```python
from build123d import *

# Parameters (mm, degrees)
SKETCH1_W           = 40
SKETCH1_H           = 40
BOSS_EXTRUDE1_DEPTH = 40
SKETCH2_W           = 10
SKETCH2_H           = 20
CUT_EXTRUDE1_DEPTH  = 40
SKETCH3_W           = 10
SKETCH3_H           = 10
CUT_EXTRUDE2_DEPTH  = 40
SKETCH4_W           = 10
SKETCH4_H           = 10
CUT_EXTRUDE4_DEPTH  = 20
SKETCH5_W           = 10
SKETCH5_H           = 10
CUT_EXTRUDE5_DEPTH  = 30


with BuildPart() as part:
    # Sketch1 → Boss-Extrude1 (new body)
    with BuildSketch(Plane.XY):
        with Locations((20, 20)):
            Rectangle(SKETCH1_W, SKETCH1_H)
    extrude(amount=BOSS_EXTRUDE1_DEPTH)

    # Sketch2 → Cut-Extrude1 (cut)
    with BuildSketch(Plane(origin=(0, 40, 0), x_dir=(1, 0, 0), z_dir=(0, 1, 0))):
        with Locations((35, -30)):
            Rectangle(SKETCH2_W, SKETCH2_H)
    extrude(amount=-CUT_EXTRUDE1_DEPTH, mode=Mode.SUBTRACT)

    # Sketch3 → Cut-Extrude2 (cut)
    with BuildSketch(Plane.ZY):
        with Locations((25, 35)):
            Rectangle(SKETCH3_W, SKETCH3_H)
        Polygon((40, 10), (40, 40), (30, 40), (30, 30), (30, 10), align=None)
    extrude(amount=-CUT_EXTRUDE2_DEPTH, mode=Mode.SUBTRACT)

    # Sketch4 → Cut-Extrude4 (cut)
    with BuildSketch(Plane(origin=(0, 30, 0), x_dir=(1, 0, 0), z_dir=(0, 1, 0))):
        with Locations((5, -25)):
            Rectangle(SKETCH4_W, SKETCH4_H)
    extrude(amount=-CUT_EXTRUDE4_DEPTH, mode=Mode.SUBTRACT)

    # Sketch5 → Cut-Extrude5 (cut)
    with BuildSketch(Plane(origin=(0, 40, 0), x_dir=(1, 0, 0), z_dir=(0, 1, 0))):
        with Locations((5, -15)):
            Rectangle(SKETCH5_W, SKETCH5_H)
    extrude(amount=-CUT_EXTRUDE5_DEPTH, mode=Mode.SUBTRACT)


solid = part.part
```
Input: part model. Units: mm. Frame: model coordinates. A direction names the side the tool comes from. Coordinates: 2 decimals unless noted, no trailing zeros. Write each loop counter-clockwise with the first axis right and the second up, starting at its lowest first coordinate (ties: lowest second). Pieces come first, ordered by that corner, then holes. Notation, with made-up numbers: (-2, 72.25) -> (54, 72.25) arc R12 cw to (54, 80.25) -> close; hole circle Ø8 at (-2, -3.5). An arc over 180 degrees is marked (long way). Write each question's results on one line, items separated by ' | '.
Item 1: Pin query (flat end, axial travel): pin 1 Ø12 at (x, z) = (29.5, 33) entering from +Y; pin 2 Ø6 at (x, y) = (10, 21) entering from +Z; pin 3 Ø12 at (x, z) = (7, 36) entering from +Y. Return the tip coordinate at first contact, or that it passes through.
Conclusion:
pin 1: stops at y = 30 | pin 2: stops at z = 30 | pin 3: stops at y = 10
Item 2: Section query B-B on x = 19.5. Return loops of the section in (y, z), plus the area to 3 significant figures.
Conclusion:
outline: (0, 0) -> (40, 0) -> (40, 20) -> (30, 20) -> (30, 30) -> (10, 30) -> (10, 40) -> (0, 40) -> close | area: 1,200 mm^2
Item 3: Section query A-A on y = 13. Return loops of the section in (x, z), plus the area to 3 significant figures.
Conclusion:
outline: (0, 0) -> (40, 0) -> (40, 20) -> (30, 20) -> (30, 30) -> (10, 30) -> (10, 10) -> (0, 10) -> close | area: 900 mm^2
Item 4: Section query D-D on y = 2.5. Return loops of the section in (x, z), plus the area to 3 significant figures.
Conclusion:
outline: (0, 0) -> (40, 0) -> (40, 20) -> (30, 20) -> (30, 40) -> (0, 40) -> close | area: 1,400 mm^2
Item 5: Set-up query: faces 1 (the flat face through (0, 11, 6)), 2 (the flat face through (15, 5, 40)), 3 (the flat face through (20, 20, 30)), 4 (the flat face through (30, 12, 28)), 5 (the flat face through (10, 22, 20)). Return all of +Z, -Z, +X, -X, +Y, -Y with unobstructed straight access to the full face (end or side cutting, diameter ignored); none if empty.
Conclusion:
face 1: +Z, -Z, -X, +Y, -Y | face 2: +Z, +X, -X, +Y, -Y | face 3: +Z, +X, -X, +Y | face 4: +Z, +X, +Y, -Y | face 5: +Z, -X, +Y
Item 6: Section query C-C on z = 17. Return loops of the section in (x, y), plus the area to 3 significant figures.
Conclusion:
outline: (0, 0) -> (40, 0) -> (40, 40) -> (10, 40) -> (10, 10) -> (0, 10) -> close | area: 1,300 mm^2
Item 7: Material intervals for probe 1 along X at (y, z) = (31, 14); probe 2 along Y at (x, z) = (3.5, 16.5), sorted ascending.
Conclusion:
probe 1: x = 10 to 40 | probe 2: y = 0 to 10
